Autodesk Inventor part; units mm, degrees
ref_plane "YZ Plane" through (0, 0, 0) normal (1, 0, 0) x (0, 1, 0)
ref_plane "XZ Plane" through (0, 0, 0) normal (0, 1, 0) x (-1, 0, 0)
ref_plane "XY Plane" through (0, 0, 0) normal (0, 0, 1) x (1, 0, 0)
sketch "Skizze1" plane through (0, 0, 0) normal (0, 0, 1) x (1, 0, 0)
  arc A0 (-4.018, -29.7297) -> (-4.018, 29.7297) centre (0, 0) ccw
  line L0 (-4.018, 29.7297) -> (-150, 10)
  line L1 (-150, 10) -> (-150, -10)
  line L2 (-150, -10) -> (-4.018, -29.7297)
  line L3 (-186, 0) -> (66, 0)
  dimension "d0" = 60
  dimension "d1" = 150
  dimension "d2" = 20
extrude "Extrusion1" add sketch "Skizze1" along normal blind 40
sketch "Skizze2" plane through (0, 0, 40) normal (0, 0, 1) x (1, 0, 0)
  line L0 (-150, 10) -> (-150, -10)
  line L1 (-150, 7.5) -> (-2.9253, 24.8283)
  arc A0 (-2.9253, -24.8283) -> (-2.9253, 24.8283) centre (0, 0) ccw
  line L2 (-150, -7.5) -> (-2.9253, -24.8283)
  line L3 (-186, 0) -> (66, 0)
  dimension "d5" = 15
  dimension "d6" = 25
extrude "Extrusion2" cut sketch "Skizze2" against normal blind 35
fillet "Rundung1" radius 7.3 3 edges at (25, 0, 5) (-76.4626, -16.1641, 5) (-76.4626, 16.1641, 5)
properties part number "Weiche_1"
Source: CAD feature listing. Evaluate the final solid. Frame: model axes, mm. A direction names the side the tool comes from. Round coordinates to 2 decimals unless told otherwise and drop trailing zeros. Order: outer loops, then holes, each group sorted by start corner. A loop starts at its lowest first (then second) coordinate and runs counter-clockwise, first axis right, second up. Notation, with made-up numbers: (17, 20.25) - (63, 20.25) arc R12 ccw to (63, 33.25) - close; hole circle Ø1 at (-39, -16). An arc over 180 degrees is marked (long way). Use a Markdown table: item, result. Add a question column.
1. First-contact query: pin 1 (1 mm diameter, centred on x = -30.5, y = 2.5, fed in from +Z); pin 2 (2 mm diameter, centred on x = -76, z = 35, fed in from +Y); pin 3 (8 mm diameter, centred on x = 11.5, y = -22.5, fed in from -Z); pin 4 (1 mm diameter, centred on x = -33.5, z = 13, fed in from -Y). Flat tips, straight axial feed; report the tip coordinate or a pass-through.
2. Section query C-C (z = 8.5). Return the cut outline in (x, y), then the cut area to 3 significant figures.
3. Mould query, pull axis X, two halves, no side actions, for faces 1 (the cylindrical face through (-75.611, -14.168, 7.195)), 2 (the flat face through (-78.031, -19.727, 19.72)), 3 (the flat face through (-41, 0, 0)). Classes: +X half, -X half, draft (parallel to the pull), parting line (faces both ways), or undercut.
4. Section query A-A (z = 24.5). Return the cut outline in (x, y).
5. Line query: probe 1 along Y at (x, z) = (0, 33); probe 2 along Z at (x, y) = (-11, -7.5); probe 3 along X at (y, z) = (0, 21). Output: solid intervals per line, ascending.
6. Set-up query: faces 4 (the flat face through (-76, 20, 20)), 5 (the flat face through (-77.492, 16.043, 26.344)). Return all of +Z, -Z, +X, -X, +Y, -Y with unobstructed straight access to the full face (end or side cutting, diameter ignored); none if empty.
7. Section query B-B (x = 0). Return the cut outline in (y, z), then the cut area to 3 significant figures.
Derived:
| question | item | result |
|---|---|---|
| 1 | pin 1 | z = 5 |
| 1 | pin 2 | y = 20.14 |
| 1 | pin 3 | z = 0 |
| 1 | pin 4 | y = -25.81 |
| 2 | outline | (-150, -10) - (-4.02, -29.73) arc R30 ccw (long way) to (-4.02, 29.73) - (-150, 10) - (-150, 6.43) - (-2.8, 23.77) arc R23.93 cw (long way) to (-2.8, -23.77) - (-150, -6.43) - close |
| 2 | area | 1,980 mm2 |
| 3 | face 1 | undercut |
| 3 | face 2 | -X half |
| 3 | face 3 | draft |
| 4 | outline | (-150, -10) - (-4.02, -29.73) arc R30 ccw (long way) to (-4.02, 29.73) - (-150, 10) - (-150, 7.5) - (-2.93, 24.83) arc R25 cw (long way) to (-2.93, -24.83) - (-150, -7.5) - close |
| 5 | probe 1 | -30 to -25, 25 to 30 |
| 5 | probe 2 | 0 to 5 |
| 5 | probe 3 | 25 to 30 |
| 6 | face 4 | +Z, -Z, -X, +Y |
| 6 | face 5 | +Z |
| 7 | outline | (-30, 0) - (30, 0) - (30, 40) - (25, 40) - (25, 12.3) arc R7.3 cw to (17.7, 5) - (-17.7, 5) arc R7.3 cw to (-25, 12.3) - (-25, 40) - (-30, 40) - close |
| 7 | area | 673 mm2 |
